from build123d import *

# Parameters (mm, degrees)
ESQUISSE1_R             = 2
TIGE_DEPTH              = 55
CHANFREIN_D_ENTR_E_SIZE = 0.7
ESQUISSE3_W             = 1
ESQUISSE3_H             = 7
FENTE_DEPTH             = 1.2


with BuildPart() as part:
    # Esquisse1 → Tige (new body)
    with BuildSketch(Plane(origin=(0, 0, 0), x_dir=(1, 0, 0), z_dir=(0, 1, 0))):
        with Locations(Location((0, 0, 0), (0, 0, 270))):
            Circle(ESQUISSE1_R)
    extrude(amount=-TIGE_DEPTH)

    # Chanfrein d_entr_e
    chanfrein_d_entr_e_edges = [part.edges().sort_by_distance(p)[0] for p in [
        (0, -55, -2),
    ]]
    chamfer(chanfrein_d_entr_e_edges, length=CHANFREIN_D_ENTR_E_SIZE)

    # Esquisse2 → T_te (revolve)
    with BuildSketch(Plane.XY, mode=Mode.PRIVATE) as t_te_sk:
        with BuildLine():
            Line((0, 0), (3.5, 0))
            Line((3.5, 0), (3.5, 2.16))
            ThreePointArc((3.5, 2.16), (3.429705627, 2.329705627), (3.26, 2.4))
            Line((3.26, 2.4), (0, 2.4))
            Line((0, 2.4), (0, 0))
        make_face()
    revolve(t_te_sk.sketch.rotate(Axis((0, 2.4, 0), (0, -1, 0)), 180), axis=Axis((0, 2.4, 0), (0, -1, 0)))

    # Esquisse3 → Fente (cut)
    with BuildSketch(Plane(origin=(0, 2.4, -1.8), x_dir=(1, 0, 0), z_dir=(0, -1, 0))):
        with Locations((0, 1.8)):
            Rectangle(ESQUISSE3_W, ESQUISSE3_H)
    extrude(amount=FENTE_DEPTH, mode=Mode.SUBTRACT)


solid = part.part
For this review, take the finished solid that the model builds, in its own axes (mm). A direction names the side the tool comes from. Give positions to 0.01 mm unless a question says otherwise; leave off trailing zeros. Loops run counter-clockwise (first coordinate to the right, second up) from the corner with the lowest first, then second, coordinate; pieces in that order, holes last. Notation, with made-up numbers: M 56,28 L 89,28 A22 ccw 89,50 Z; hole C 54.5,50 d4. An arc over 180 degrees is marked long. Put each result on its own line as item: value. Start each with the question number.
(1) For pin 1 (1.1 mm diameter, centred on x = 0, z = -1, fed in from +Y); pin 2 (1.5 mm diameter, centred on x = -1, y = -6.5, fed in from +Z); pin 3 (1.3 mm diameter, centred on y = 2, z = -1, fed in from -X); pin 4 (1.5 mm diameter, centred on x = 0.5, z = -2.5, fed in from -Y), all flat-tipped, find the tip position at first contact; note any pin that passes through.
(2) Wall thickness on L1, parallel to Y at x = 0.25, z = 0.25; L2, parallel to Y at x = -2, z = -1.5; L3, parallel to X at y = -17, z = 0: over which ranges is each line inside the solid? List them lowest first.
(3) Add section B-B, the plane x = 0. Write out the cut boundary in (y, z).
(4) Add section C-C, the plane y = -5. Write out the cut boundary in (x, z).
(5) Add section A-A, the plane z = 0. Write out the cut boundary in (x, y), then the cut area to 3 significant figures.
(6) Machinability: for faces 1 (the flat face through (0.5, 2, 0)), 2 (the flat face through (2, 0, 2)), 3 (the cylindrical face through (-1.615, 1.095, 3.105)), which of the approach directions +Z, -Z, +X, -X, +Y, -Y give a long, thin tool a straight path to every point of the face, cutting with its end or side? Answer none if there is none.
Result:
1. pin 1: stops at y = 2.4
1. pin 2: stops at z = 1.98
1. pin 3: stops at x = -3.48
1. pin 4: stops at y = -54.5
2. L1: y = -55 to 1.2
2. L2: y = 0 to 2.4
2. L3: x = -2 to 2
3. outline: M -55,-1.3 L -54.3,-2 L 0,-2 L 0,-3.5 L 1.2,-3.5 L 1.2,3.5 L 0,3.5 L 0,2 L -54.3,2 L -55,1.3 Z
4. outline: C 0,0 d4
5. outline: M -3.5,0 L -2,0 L -2,-54.3 L -1.3,-55 L 1.3,-55 L 2,-54.3 L 2,0 L 3.5,0 L 3.5,2.16 A0.24 ccw 3.26,2.4 L 0.5,2.4 L 0.5,1.2 L -0.5,1.2 L -0.5,2.4 L -3.26,2.4 A0.24 ccw -3.5,2.16 Z
5. area: 235 mm^2
6. face 1: +Z, -Z, +Y
6. face 2: -Y
6. face 3: +Y, -Y
